from build123d import *

# Parameters (mm, degrees)
F0_R     = 2
F1_DEPTH = 10
F2_DEPTH = 11
F3_DEPTH = 1


# Not quite as in the source:
# - a fillet or chamfer that OpenCascade refuses, or shapes differently, is made with other operations: its cross-section is extruded or revolved along the edge and cut away or added
# - after a boolean that leaves OpenCascade's solid faulty, fix() repairs it


with BuildPart() as f1:
    # F0 (on Top) → F1 (new body)
    with BuildSketch(Plane.XY):
        with BuildLine():
            Line((26, 0), (6, 0))
            ThreePointArc((6, 0), (3.3334213981, -4.9888176738), (-2.2961005942, -5.5432771951))
            Line((-2.2961005942, -5.5432771951), (52.3313164038, -28.170694193))
            ThreePointArc((52.3313164038, -28.170694193), (48.7427053156, -23.7979589301), (50.3847763109, -18.3847763109))
            Line((50.3847763109, -18.3847763109), (36.2426406871, -4.2426406871))
            ThreePointArc((36.2426406871, -4.2426406871), (29.7038994058, -5.5432771951), (26, 0))
        make_face()
        with BuildLine():
            ThreePointArc((0, 6), (4.2426406871, 4.2426406871), (6, 0))
            Line((6, 0), (26, 0))
            ThreePointArc((26, 0), (27.7573593129, 4.2426406871), (32, 6))
            Line((32, 6), (0, 6))
        make_face()
        with BuildLine():
            ThreePointArc((38, 0), (37.5432771951, -2.2961005942), (36.2426406871, -4.2426406871))
            Line((36.2426406871, -4.2426406871), (50.3847763109, -18.3847763109))
            ThreePointArc((50.3847763109, -18.3847763109), (54.627416998, -16.627416998), (58.8700576851, -18.3847763109))
            Line((58.8700576851, -18.3847763109), (36.2426406871, 4.2426406871))
            ThreePointArc((36.2426406871, 4.2426406871), (37.5432771951, 2.2961005942), (38, 0))
        make_face()
        with BuildLine():
            ThreePointArc((-2.2961005942, -5.5432771951), (3.3334213981, -4.9888176738), (6, 0))
            ThreePointArc((6, 0), (4.2426406871, 4.2426406871), (0, 6))
            ThreePointArc((0, 6), (-5.8847116824, 1.1705419321), (-2.2961005942, -5.5432771951))
        make_face()
        Circle(F0_R, mode=Mode.SUBTRACT)
        with BuildLine():
            Line((30, 0), (26, 0))
            ThreePointArc((26, 0), (29.7038994058, -5.5432771951), (36.2426406871, -4.2426406871))
            Line((36.2426406871, -4.2426406871), (33.4142135624, -1.4142135624))
            ThreePointArc((33.4142135624, -1.4142135624), (31.2346331353, -1.847759065), (30, 0))
        make_face()
        with BuildLine():
            ThreePointArc((32, 6), (27.7573593129, 4.2426406871), (26, 0))
            Line((26, 0), (30, 0))
            ThreePointArc((30, 0), (32, 2), (34, 0))
            ThreePointArc((34, 0), (33.847759065, -0.7653668647), (33.4142135624, -1.4142135624))
            Line((33.4142135624, -1.4142135624), (36.2426406871, -4.2426406871))
            ThreePointArc((36.2426406871, -4.2426406871), (37.5432771951, -2.2961005942), (38, 0))
            ThreePointArc((38, 0), (37.5432771951, 2.2961005942), (36.2426406871, 4.2426406871))
            ThreePointArc((36.2426406871, 4.2426406871), (34.2961005942, 5.5432771951), (32, 6))
        make_face()
        with BuildLine():
            ThreePointArc((50.3847763109, -18.3847763109), (48.7427053156, -23.7979589301), (52.3313164038, -28.170694193))
            ThreePointArc((52.3313164038, -28.170694193), (57.9608383961, -27.6162346718), (60.627416998, -22.627416998))
            ThreePointArc((60.627416998, -22.627416998), (60.170694193, -20.3313164038), (58.8700576851, -18.3847763109))
            ThreePointArc((58.8700576851, -18.3847763109), (54.627416998, -16.627416998), (50.3847763109, -18.3847763109))
        make_face()
        with BuildLine():
            ThreePointArc((56.627416998, -22.627416998), (53.8620501332, -24.475176063), (53.2132034356, -21.2132034356))
            ThreePointArc((53.2132034356, -21.2132034356), (55.3927838627, -20.7796579329), (56.627416998, -22.627416998))
        make_face(mode=Mode.SUBTRACT)
    extrude(amount=F1_DEPTH)

    # F0 (on Top) → F2 (join)
    with BuildSketch(Plane.XY):
        with BuildLine():
            ThreePointArc((-2.2961005942, -5.5432771951), (3.3334213981, -4.9888176738), (6, 0))
            ThreePointArc((6, 0), (4.2426406871, 4.2426406871), (0, 6))
            ThreePointArc((0, 6), (-5.8847116824, 1.1705419321), (-2.2961005942, -5.5432771951))
        make_face()
        Circle(F0_R, mode=Mode.SUBTRACT)
        with BuildLine():
            ThreePointArc((32, 6), (27.7573593129, 4.2426406871), (26, 0))
            Line((26, 0), (30, 0))
            ThreePointArc((30, 0), (32, 2), (34, 0))
            ThreePointArc((34, 0), (33.847759065, -0.7653668647), (33.4142135624, -1.4142135624))
            Line((33.4142135624, -1.4142135624), (36.2426406871, -4.2426406871))
            ThreePointArc((36.2426406871, -4.2426406871), (37.5432771951, -2.2961005942), (38, 0))
            ThreePointArc((38, 0), (37.5432771951, 2.2961005942), (36.2426406871, 4.2426406871))
            ThreePointArc((36.2426406871, 4.2426406871), (34.2961005942, 5.5432771951), (32, 6))
        make_face()
        with BuildLine():
            Line((30, 0), (26, 0))
            ThreePointArc((26, 0), (29.7038994058, -5.5432771951), (36.2426406871, -4.2426406871))
            Line((36.2426406871, -4.2426406871), (33.4142135624, -1.4142135624))
            ThreePointArc((33.4142135624, -1.4142135624), (31.2346331353, -1.847759065), (30, 0))
        make_face()
        with BuildLine():
            ThreePointArc((50.3847763109, -18.3847763109), (48.7427053156, -23.7979589301), (52.3313164038, -28.170694193))
            ThreePointArc((52.3313164038, -28.170694193), (57.9608383961, -27.6162346718), (60.627416998, -22.627416998))
            ThreePointArc((60.627416998, -22.627416998), (60.170694193, -20.3313164038), (58.8700576851, -18.3847763109))
            ThreePointArc((58.8700576851, -18.3847763109), (54.627416998, -16.627416998), (50.3847763109, -18.3847763109))
        make_face()
        with BuildLine():
            ThreePointArc((56.627416998, -22.627416998), (53.8620501332, -24.475176063), (53.2132034356, -21.2132034356))
            ThreePointArc((53.2132034356, -21.2132034356), (55.3927838627, -20.7796579329), (56.627416998, -22.627416998))
        make_face(mode=Mode.SUBTRACT)
    extrude(amount=F2_DEPTH)

    # F0 (on Top) → F3 (join)
    with BuildSketch(Plane.XY):
        with BuildLine():
            ThreePointArc((-2.2961005942, -5.5432771951), (3.3334213981, -4.9888176738), (6, 0))
            ThreePointArc((6, 0), (4.2426406871, 4.2426406871), (0, 6))
            ThreePointArc((0, 6), (-5.8847116824, 1.1705419321), (-2.2961005942, -5.5432771951))
        make_face()
        Circle(F0_R, mode=Mode.SUBTRACT)
        with BuildLine():
            ThreePointArc((32, 6), (27.7573593129, 4.2426406871), (26, 0))
            Line((26, 0), (30, 0))
            ThreePointArc((30, 0), (32, 2), (34, 0))
            ThreePointArc((34, 0), (33.847759065, -0.7653668647), (33.4142135624, -1.4142135624))
            Line((33.4142135624, -1.4142135624), (36.2426406871, -4.2426406871))
            ThreePointArc((36.2426406871, -4.2426406871), (37.5432771951, -2.2961005942), (38, 0))
            ThreePointArc((38, 0), (37.5432771951, 2.2961005942), (36.2426406871, 4.2426406871))
            ThreePointArc((36.2426406871, 4.2426406871), (34.2961005942, 5.5432771951), (32, 6))
        make_face()
        with BuildLine():
            Line((30, 0), (26, 0))
            ThreePointArc((26, 0), (29.7038994058, -5.5432771951), (36.2426406871, -4.2426406871))
            Line((36.2426406871, -4.2426406871), (33.4142135624, -1.4142135624))
            ThreePointArc((33.4142135624, -1.4142135624), (31.2346331353, -1.847759065), (30, 0))
        make_face()
        with BuildLine():
            ThreePointArc((50.3847763109, -18.3847763109), (48.7427053156, -23.7979589301), (52.3313164038, -28.170694193))
            ThreePointArc((52.3313164038, -28.170694193), (57.9608383961, -27.6162346718), (60.627416998, -22.627416998))
            ThreePointArc((60.627416998, -22.627416998), (60.170694193, -20.3313164038), (58.8700576851, -18.3847763109))
            ThreePointArc((58.8700576851, -18.3847763109), (54.627416998, -16.627416998), (50.3847763109, -18.3847763109))
        make_face()
        with BuildLine():
            ThreePointArc((56.627416998, -22.627416998), (53.8620501332, -24.475176063), (53.2132034356, -21.2132034356))
            ThreePointArc((53.2132034356, -21.2132034356), (55.3927838627, -20.7796579329), (56.627416998, -22.627416998))
        make_face(mode=Mode.SUBTRACT)
    extrude(amount=-F3_DEPTH)

    add(f1.part.fix(), mode=Mode.REPLACE)

    # F4: chamfer of 1 on 6 edges, made by hand

    # F4_s1 → F4_t2 (revolve, cut)
    with BuildSketch(Plane.XZ):
        Polygon((3, 11), (2, 10), (2, 11), align=None)
    revolve(axis=Axis((0, 0, 11), (0, 0, 1)), mode=Mode.SUBTRACT)

    # F4_s3 → F4_t4 (revolve, cut)
    with BuildSketch(Plane(origin=(16, 16, 0), x_dir=(0, 0, 1), z_dir=(0.7071067812, 0.7071067812, 0))):
        Polygon((11, 25.627416998), (10, 24.627416998), (11, 24.627416998), align=None)
    revolve(axis=Axis((32, 0, 11), (0, 0, -1)), mode=Mode.SUBTRACT)

    # F4_s5 → F4_t6 (revolve, cut)
    with BuildSketch(Plane(origin=(16, 16, 0), x_dir=(0, 0, 1), z_dir=(-0.7071067812, -0.7071067812, 0))):
        Polygon((11, -51.627416998), (10, -52.627416998), (11, -52.627416998), align=None)
    revolve(axis=Axis((54.627416998, -22.627416998, 11), (0, 0, -1)), mode=Mode.SUBTRACT)

    # F4_s7 → F4_t8 (revolve, cut)
    with BuildSketch(Plane.XZ):
        Polygon((3, -1), (2, 0), (2, -1), align=None)
    revolve(axis=Axis((0, 0, -1), (0, 0, 1)), mode=Mode.SUBTRACT)

    # F4_s9 → F4_t10 (revolve, cut)
    with BuildSketch(Plane(origin=(16, 16, 0), x_dir=(0, 0, 1), z_dir=(0.7071067812, 0.7071067812, 0))):
        Polygon((-1, 25.627416998), (0, 24.627416998), (-1, 24.627416998), align=None)
    revolve(axis=Axis((32, 0, -1), (0, 0, -1)), mode=Mode.SUBTRACT)

    # F4_s11 → F4_t12 (revolve, cut)
    with BuildSketch(Plane(origin=(16, 16, 0), x_dir=(0, 0, 1), z_dir=(-0.7071067812, -0.7071067812, 0))):
        Polygon((-1, -51.627416998), (0, -52.627416998), (-1, -52.627416998), align=None)
    revolve(axis=Axis((54.627416998, -22.627416998, -1), (0, 0, -1)), mode=Mode.SUBTRACT)


solid = f1.part
Here's how the part is built. I have some questions about the finished solid (model axes, mm). Round coordinates to 2 decimals unless told otherwise and drop trailing zeros. Order: outer loops, then holes, each group sorted by start corner. A loop starts at its lowest first (then second) coordinate and runs counter-clockwise, first axis right, second up. Notation, with made-up numbers: (-29, -11) -> (-9, -11) arc R21 ccw to (-9, 19) -> close; hole circle Ø5 at (78, 66.5). An arc over 180 degrees is marked (long way). Return JSON: item names as keys, results as strings.
Q1. I need wall thicknesses on line 1 along Y through (x, z) = (0, 3); line 2 along Z through (x, y) = (55, -16); line 3 along Y through (x, z) = (55.5, 0.25). Which ranges of each line are inside material? Lowest first, please. Write a range as from..to.
Filled sheet:
{"line 1": "y = -6.49..-2, 2..6", "line 2": "z = 0..10", "line 3": "y = -28.56..-24.43, -20.83..-15.01"}
Q2. For pin 1 Ø5 at (x, z) = (30, 3.5) entering from -Y; pin 2 Ø4.5 at (x, y) = (32, 0) entering from +Z; pin 3 Ø1 at (y, z) = (-15.5, 5) entering from -X, each with a flat end and sliding along its axis, tell me the tip position at first contact or that it passes through.
Filled sheet:
{"pin 1": "stops at y = -19.96", "pin 2": "stops at z = 10.25", "pin 3": "stops at x = 20.53"}
Q3. If we section it at A-A on z = 3.5: List the corners of the cut face in (x, y) for me.
Filled sheet:
{"outline": "(-2.3, -5.54) -> (52.33, -28.17) arc R6 ccw to (58.87, -18.38) -> (36.24, 4.24) arc R6 ccw to (32, 6) -> (0, 6) arc R6 ccw to start; hole circle Ø4 at (0, 0); hole circle Ø4 at (32, 0); hole circle Ø4 at (54.63, -22.63)"}
Q4. If we section it at C-C on y = -11.5: List the corners of the cut face in (x, z) for me, plus the area to 3 significant figures.
Filled sheet:
{"outline": "(12.08, 0) -> (51.99, 0) -> (51.99, 10) -> (12.08, 10) -> close", "area": "399 mm^2"}
Q5. If we mould it in two halves opening along X, with no side actions, what happens to faces 1 (the cylindrical face through (33.908, -0.601, 4.93)), 2 (the flat face through (24.64, -16.7, 4.93)), 3 (the flat face through (57, -25, 11))? For each: released by +X, released by -X, zero draft, split by the parting line, or undercut.
Filled sheet:
{"face 1": "undercut", "face 2": "released by -X", "face 3": "zero draft"}
Q6. If we section it at B-B on x = 25: List the corners of the cut face in (y, z) for me, plus the area to 3 significant figures.
Filled sheet:
{"outline": "(-16.85, 0) -> (6, 0) -> (6, 10) -> (-16.85, 10) -> close", "area": "228 mm^2"}
